Geometry: final body of the model. Coordinates: model frame, mm. Face numbers are marked on the shaded views. A direction names the side the tool comes from. Give positions to 0.01 mm unless a question says otherwise; leave off trailing zeros. Write each loop counter-clockwise with the first axis right and the second up, starting at its lowest first coordinate (ties: lowest second). Pieces come first, ordered by that corner, then holes. Notation, with made-up numbers: (-39.5, 4) -> (0.5, 4) arc R18 ccw to (0.5, 23) -> close; hole circle Ø9 at (54, 27.5). An arc over 180 degrees is marked (long way). Answer in a Markdown table with one row per item. Add a question column.
Item 1: First-contact query: P1, Ø1.5, axis at x = 57, z = 0.5, coming from the +Y side. Flat tip, straight axial feed; report the tip coordinate or a pass-through.
Item 2: Material intervals for probe 1 along Z at (x, y) = (58, 4.2); probe 2 along Z at (x, y) = (67.5, 3.2); probe 3 along Z at (x, y) = (47.5, 3.9), sorted ascending. Write a range as from..to.
Item 3: Section query D-D on x = 60. Output: boundary loops of the cut face in (y, z).
Item 4: Section query C-C on y = 3. Output: boundary loops of the cut face in (x, z), plus the area to 3 significant figures.
Item 5: Access query for the marked faces 1 and 2. Directions: +Z, -Z, +X, -X, +Y, -Y. A direction counts if a zero-diameter tool reaches every point of the face in a straight line with its end or side. Return the directions, or none.
Item 6: Section query B-B on z = -0.5. Output: boundary loops of the cut face in (x, y).
Item 7: Section query A-A on x = 73.5. Output: boundary loops of the cut face in (y, z).
Item 8: Draft query along X for the marked faces 3 and 4. Return one class per face: +X half, -X half, draft (parallel to the pull), parting line (faces both ways), or undercut.
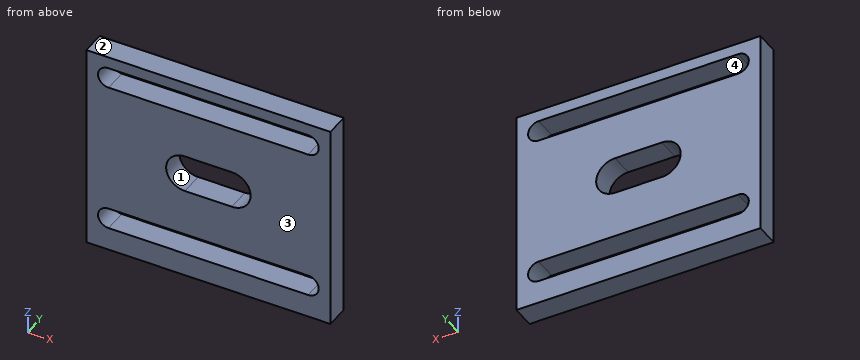
```python
from build123d import *

# Parameters (mm, degrees)
SKETCH1_R           = 4
BOSS_EXTRUDE1_DEPTH = 5
CUT_EXTRUDE1_DEPTH  = 10
CUT_EXTRUDE2_DEPTH  = 10
CUT_EXTRUDE5_START  = -75
SKETCH5_R           = 1.6
CUT_EXTRUDE5_DEPTH  = 10
SKETCH6_W           = 85
SKETCH6_H           = 75
CUT_EXTRUDE6_DEPTH  = 10
SKETCH7_W           = 65
SKETCH7_H           = 15
CUT_EXTRUDE7_DEPTH  = 10
SKETCH8_W           = 12.986544032
SKETCH8_H           = 50
CUT_EXTRUDE8_DEPTH  = 10
SKETCH9_W           = 52.013455968
SKETCH9_H           = 5.5
CUT_EXTRUDE9_DEPTH  = 10


with BuildPart() as part:
    # Sketch1 → Boss-Extrude1 (new body)
    with BuildSketch(Plane(origin=(0, 0, 0), x_dir=(1, 0, 0), z_dir=(0, 1, 0))):
        with BuildLine():
            Line((-57.373232891, 17.353168425), (-57.373232891, -35.646831575))
            Line((-57.373232891, -35.646831575), (-57.373232891, -43.646831575))
            Line((-57.373232891, -43.646831575), (92.626767109, -43.646831575))
            Line((92.626767109, -43.646831575), (92.626767109, -35.646831575))
            Line((92.626767109, -35.646831575), (92.626767109, 29.353168425))
            ThreePointArc((92.626767109, 29.353168425), (92.040980672, 30.767381987), (90.626767109, 31.353168425))
            Line((90.626767109, 31.353168425), (26.626767109, 31.353168425))
            Line((26.626767109, 31.353168425), (-57.373232891, 31.353168425))
            Line((-57.373232891, 31.353168425), (-57.373232891, 17.353168425))
        make_face()
        with Locations((-25.373232891, -2.646831575)):
            Circle(SKETCH1_R, mode=Mode.SUBTRACT)
        with BuildLine():
            Line((32.363311142, 16.366624392), (74.890223077, 16.366624392))
            ThreePointArc((74.890223077, 16.366624392), (77.140223077, 14.116624392), (74.890223077, 11.866624392))
            Line((74.890223077, 11.866624392), (32.363311142, 11.866624392))
            ThreePointArc((32.363311142, 11.866624392), (30.113311142, 14.116624392), (32.363311142, 16.366624392))
        make_face(mode=Mode.SUBTRACT)
        with BuildLine():
            Line((32.363311142, -20.660287542), (74.890223077, -20.660287542))
            ThreePointArc((74.890223077, -20.660287542), (77.140223077, -18.410287542), (74.890223077, -16.160287542))
            Line((74.890223077, -16.160287542), (32.363311142, -16.160287542))
            ThreePointArc((32.363311142, -16.160287542), (30.113311142, -18.410287542), (32.363311142, -20.660287542))
        make_face(mode=Mode.SUBTRACT)
        with BuildLine():
            Line((48.626767109, 1.853168425), (58.626767109, 1.853168425))
            ThreePointArc((58.626767109, 1.853168425), (62.626767109, -2.146831575), (58.626767109, -6.146831575))
            Line((58.626767109, -6.146831575), (48.626767109, -6.146831575))
            ThreePointArc((48.626767109, -6.146831575), (44.626767109, -2.146831575), (48.626767109, 1.853168425))
        make_face(mode=Mode.SUBTRACT)
    extrude(amount=BOSS_EXTRUDE1_DEPTH)

    # Sketch2 → Cut-Extrude1 (cut)
    with BuildSketch(Plane(origin=(0, 5, 0), x_dir=(1, 0, 0), z_dir=(0, 1, 0))):
        with BuildLine():
            Line((-47.394048171, 11.623983705), (-13.35241761, 11.623983705))
            ThreePointArc((-13.35241761, 11.623983705), (-11.10241761, 9.373983705), (-13.35241761, 7.123983705))
            Line((-13.35241761, 7.123983705), (-47.394048171, 7.123983705))
            ThreePointArc((-47.394048171, 7.123983705), (-49.644048171, 9.373983705), (-47.394048171, 11.623983705))
        make_face()
        with BuildLine():
            Line((-47.394048171, -16.917646855), (-13.35241761, -16.917646855))
            ThreePointArc((-13.35241761, -16.917646855), (-11.10241761, -14.667646855), (-13.35241761, -12.417646855))
            Line((-13.35241761, -12.417646855), (-47.394048171, -12.417646855))
            ThreePointArc((-47.394048171, -12.417646855), (-49.644048171, -14.667646855), (-47.394048171, -16.917646855))
        make_face()
        with BuildLine():
            Line((-35.373232891, 1.353168425), (-25.373232891, 1.353168425))
            ThreePointArc((-25.373232891, 1.353168425), (-21.373232891, -2.646831575), (-25.373232891, -6.646831575))
            Line((-25.373232891, -6.646831575), (-35.373232891, -6.646831575))
            ThreePointArc((-35.373232891, -6.646831575), (-39.373232891, -2.646831575), (-35.373232891, 1.353168425))
        make_face()
    extrude(amount=-CUT_EXTRUDE1_DEPTH, mode=Mode.SUBTRACT)

    # Sketch3 → Cut-Extrude2 (cut)
    with BuildSketch(Plane(origin=(0, 5, 0), x_dir=(1, 0, 0), z_dir=(0, 1, 0))):
        with BuildLine():
            Line((21.749403979, 13.353168425), (21.749403979, 3.353168425))
            ThreePointArc((21.749403979, 3.353168425), (17.749403979, -0.646831575), (13.749403979, 3.353168425))
            Line((13.749403979, 3.353168425), (13.749403979, 13.353168425))
            ThreePointArc((13.749403979, 13.353168425), (17.749403979, 17.353168425), (21.749403979, 13.353168425))
        make_face()
        with BuildLine():
            Line((21.749403979, -14.646831575), (21.749403979, -24.646831575))
            ThreePointArc((21.749403979, -24.646831575), (17.749403979, -28.646831575), (13.749403979, -24.646831575))
            Line((13.749403979, -24.646831575), (13.749403979, -14.646831575))
            ThreePointArc((13.749403979, -14.646831575), (17.749403979, -10.646831575), (21.749403979, -14.646831575))
        make_face()
    extrude(amount=-CUT_EXTRUDE2_DEPTH, mode=Mode.SUBTRACT)

    # Sketch5 → Cut-Extrude5 (cut)
    with BuildSketch(Plane.XY.offset(43.646831575).offset(CUT_EXTRUDE5_START)):
        with Locations((-47.373232891, 2.5)):
            Circle(SKETCH5_R)
        with Locations((82.626767109, 2.5)):
            Circle(SKETCH5_R)
    extrude(amount=CUT_EXTRUDE5_DEPTH, mode=Mode.SUBTRACT)

    # Sketch6 → Cut-Extrude6 (cut)
    with BuildSketch(Plane(origin=(0, 5, 0), x_dir=(1, 0, 0), z_dir=(0, 1, 0))):
        with Locations((-14.873232891, -6.146831575)):
            Rectangle(SKETCH6_W, SKETCH6_H)
    extrude(amount=-CUT_EXTRUDE6_DEPTH, mode=Mode.SUBTRACT)

    # Sketch7 → Cut-Extrude7 (cut)
    with BuildSketch(Plane(origin=(0, 5, 0), x_dir=(1, 0, 0), z_dir=(0, 1, 0))):
        with Locations((60.126767109, -36.146831575)):
            Rectangle(SKETCH7_W, SKETCH7_H)
    extrude(amount=-CUT_EXTRUDE7_DEPTH, mode=Mode.SUBTRACT)

    # Sketch8 → Cut-Extrude8 (cut)
    with BuildSketch(Plane(origin=(0, 5, 0), x_dir=(1, 0, 0), z_dir=(0, 1, 0))):
        with BuildLine():
            Line((90.626767109, 31.353168425), (27.626767109, 31.353168425))
            Line((27.626767109, 31.353168425), (27.626767109, 21.353168425))
            Line((27.626767109, 21.353168425), (79.640223077, 21.353168425))
            Line((79.640223077, 21.353168425), (92.626767109, 21.353168425))
            Line((92.626767109, 21.353168425), (92.626767109, 29.353168425))
            ThreePointArc((92.626767109, 29.353168425), (92.040980672, 30.767381987), (90.626767109, 31.353168425))
        make_face()
        with Locations((86.133495093, -3.646831575)):
            Rectangle(SKETCH8_W, SKETCH8_H)
    extrude(amount=-CUT_EXTRUDE8_DEPTH, mode=Mode.SUBTRACT)

    # Sketch9 → Cut-Extrude9 (cut)
    with BuildSketch(Plane(origin=(0, 5, 0), x_dir=(1, 0, 0), z_dir=(0, 1, 0))):
        with Locations((53.633495093, -25.896831575)):
            Rectangle(SKETCH9_W, SKETCH9_H)
    extrude(amount=-CUT_EXTRUDE9_DEPTH, mode=Mode.SUBTRACT)


solid = part.part
```
Findings below:
| question | item | result |
|---|---|---|
| 1 | P1 | passes through |
| 2 | probe 1 | z = -21.35..-16.37, -11.87..-1.85, 6.15..16.16, 20.66..23.15 |
| 2 | probe 2 | z = -21.35..-16.37, -11.87..16.16, 20.66..23.15 |
| 2 | probe 3 | z = -21.35..-16.37, -11.87..-1.69, 5.98..16.16, 20.66..23.15 |
| 3 | outline | (0, -21.35) -> (5, -21.35) -> (5, -16.37) -> (0, -16.37) -> close; (0, -11.87) -> (5, -11.87) -> (5, -1.61) -> (0, -1.61) -> close; (0, 5.9) -> (5, 5.9) -> (5, 16.16) -> (0, 16.16) -> close; (0, 20.66) -> (5, 20.66) -> (5, 23.15) -> (0, 23.15) -> close |
| 4 | outline | (27.63, -21.35) -> (79.64, -21.35) -> (79.64, 23.15) -> (27.63, 23.15) -> close; hole (32.36, -16.37) -> (74.89, -16.37) arc R2.25 ccw to (74.89, -11.87) -> (32.36, -11.87) arc R2.25 ccw to start; hole (32.36, 16.16) -> (74.89, 16.16) arc R2.25 ccw to (74.89, 20.66) -> (32.36, 20.66) arc R2.25 ccw to start; hole (48.63, -1.85) -> (58.63, -1.85) arc R4 ccw to (58.63, 6.15) -> (48.63, 6.15) arc R4 ccw to start |
| 4 | area | 1,770 mm^2 |
| 5 | face 1 | +Y, -Y |
| 5 | face 2 | +Z, +X, -X, +Y, -Y |
| 6 | outline | (27.63, 0) -> (45.63, 0) -> (45.63, 5) -> (27.63, 5) -> close; (61.63, 0) -> (79.64, 0) -> (79.64, 5) -> (61.63, 5) -> close |
| 7 | outline | (0, -21.35) -> (5, -21.35) -> (5, -16.37) -> (0, -16.37) -> close; (0, -11.87) -> (5, -11.87) -> (5, 16.16) -> (0, 16.16) -> close; (0, 20.66) -> (5, 20.66) -> (5, 23.15) -> (0, 23.15) -> close |
| 8 | face 3 | draft |
| 8 | face 4 | undercut |
